```python
from build123d import *

# Parameters (mm, degrees)
SKETCH1_W           = 24.726477024
SKETCH1_H           = 15
SKETCH1_W_2         = 30
SKETCH1_H_2         = 20
BOSS_EXTRUDE1_DEPTH = 15
SKETCH1_4_W         = 24.726477024
SKETCH1_4_H         = 15
BOSS_EXTRUDE2_DEPTH = 40
SKETCH1_5_W         = 24.726477024
SKETCH1_5_H         = 15
CUT_EXTRUDE1_DEPTH  = 40
SKETCH1_6_W         = 30
SKETCH1_6_H         = 20
CUT_EXTRUDE2_DEPTH  = 40


with BuildPart() as part:
    # Sketch1 → Boss-Extrude1 (new body)
    with BuildSketch(Plane(origin=(0, 0, 0), x_dir=(1, 0, 0), z_dir=(0, 1, 0))):
        with Locations((-37.636761488, 22.5)):
            Rectangle(SKETCH1_W, SKETCH1_H)
        Polygon((25.273522976, 30), (-25.273522976, 30), (-25.273522976, 15), (-50, 15), (-50, -15), (-25.273522976, -15), (-25.273522976, -30), (25.273522976, -30), (25.273522976, -15), (50, -15), (50, 15), (25.273522976, 15), align=None)
        Rectangle(SKETCH1_W_2, SKETCH1_H_2, mode=Mode.SUBTRACT)
        Rectangle(SKETCH1_W_2, SKETCH1_H_2)
        with Locations((37.636761488, 22.5)):
            Rectangle(SKETCH1_W, SKETCH1_H)
        with Locations((37.636761488, -22.5)):
            Rectangle(SKETCH1_W, SKETCH1_H)
        with Locations((-37.636761488, -22.5)):
            Rectangle(SKETCH1_W, SKETCH1_H)
    extrude(amount=BOSS_EXTRUDE1_DEPTH)

    # Sketch1_4 → Boss-Extrude2 (add)
    with BuildSketch(Plane(origin=(0, 0, 0), x_dir=(1, 0, 0), z_dir=(0, 1, 0))):
        with Locations((-37.636761488, 22.5)):
            Rectangle(SKETCH1_4_W, SKETCH1_4_H)
        with Locations((37.636761488, -22.5)):
            Rectangle(SKETCH1_4_W, SKETCH1_4_H)
    extrude(amount=BOSS_EXTRUDE2_DEPTH)

    # Sketch1_5 → Cut-Extrude1 (cut)
    with BuildSketch(Plane(origin=(0, 0, 0), x_dir=(1, 0, 0), z_dir=(0, 1, 0))):
        with Locations((-37.636761488, -22.5)):
            Rectangle(SKETCH1_5_W, SKETCH1_5_H)
        with Locations((37.636761488, 22.5)):
            Rectangle(SKETCH1_5_W, SKETCH1_5_H)
    extrude(amount=CUT_EXTRUDE1_DEPTH, mode=Mode.SUBTRACT)

    # Sketch1_6 → Cut-Extrude2 (cut)
    with BuildSketch(Plane(origin=(0, 0, 0), x_dir=(1, 0, 0), z_dir=(0, 1, 0))):
        Rectangle(SKETCH1_6_W, SKETCH1_6_H)
    extrude(amount=CUT_EXTRUDE2_DEPTH, mode=Mode.SUBTRACT)


solid = part.part
```
Verification items for the finished model (mm, model axes). A direction names the side the tool comes from. Coordinates: 2 decimals unless noted, no trailing zeros. Loops run counter-clockwise (first coordinate to the right, second up) from the corner with the lowest first, then second, coordinate; pieces in that order, holes last. Notation, with made-up numbers: (38.25, 39.25) -> (94.25, 39.25) arc R18 ccw to (94.25, 70.25) -> close; hole circle Ø3 at (22, 85.5). An arc over 180 degrees is marked (long way). Answer in a Markdown table with one row per item. Add a question column.
1. Depth check by flat-ended pin: P1, Ø12, axis at x = -3, z = -22, coming from the -Y side; P2, Ø12, axis at y = 33.5, z = 20, coming from the -X side; P3, Ø12.5, axis at x = 40, y = 27, coming from the -Z side; P4, Ø12.5, axis at x = -32, y = 21.5, coming from the +Z side. Enter the tip coordinate at first touch or a pass-through.
2. Section check A-A, the plane z = 7. Enter the section's corners in (x, y), then the cut area to 3 significant figures.
3. Section check C-C, the plane x = -9.5. Enter the section's corners in (y, z), then the cut area to 3 significant figures.
4. Material ranges on probe 1 along Z at (x, y) = (-13, 11); probe 2 along X at (y, z) = (9, -7); probe 3 along X at (y, z) = (12.5, 28.5), recorded low to high. Write a range as [from, to].
5. Access from +Z, -Z, +X, -X, +Y, -Y to the whole of each face (thin tool, end or side, straight path). Record for faces 1 (the face through (0, 7, -10)), 2 (the face through (25.274, 7, -22)), 3 (the face through (25.274, 27, 23)), 4 (the face through (-25.274, 7, 23)), 5 (the face through (-25.274, 27, -22)).
6. Section check D-D, the plane z = -16.5. Enter the section's corners in (x, y).
7. Section check B-B, the plane y = 8. Enter the section's corners in (x, z).
Derived:
| question | item | result |
|---|---|---|
| 1 | P1 | stops at y = 0 |
| 1 | P2 | stops at x = 25.27 |
| 1 | P3 | stops at z = 15 |
| 1 | P4 | stops at z = -15 |
| 2 | outline | (-50, 0) -> (-15, 0) -> (-15, 15) -> (-50, 15) -> close; (15, 0) -> (50, 0) -> (50, 15) -> (15, 15) -> close |
| 2 | area | 1,050 mm² |
| 3 | outline | (0, -30) -> (15, -30) -> (15, -10) -> (0, -10) -> close; (0, 10) -> (15, 10) -> (15, 30) -> (0, 30) -> close |
| 3 | area | 600 mm² |
| 4 | probe 1 | z = [-30, -10], [10, 30] |
| 4 | probe 2 | x = [-50, -15], [15, 50] |
| 4 | probe 3 | x = [-25.27, 50] |
| 5 | face 1 | +Y, -Y |
| 5 | face 2 | -Z, +X, +Y, -Y |
| 5 | face 3 | +Z, -Z, -X, +Y |
| 5 | face 4 | +Z, -X, +Y, -Y |
| 5 | face 5 | +Z, -Z, +X, +Y |
| 6 | outline | (-50, 0) -> (25.27, 0) -> (25.27, 15) -> (-25.27, 15) -> (-25.27, 40) -> (-50, 40) -> close |
| 7 | outline | (-50, -30) -> (25.27, -30) -> (25.27, -15) -> (50, -15) -> (50, 30) -> (-25.27, 30) -> (-25.27, 15) -> (-50, 15) -> close; hole (-15, -10) -> (15, -10) -> (15, 10) -> (-15, 10) -> close |
